Could you check a few things on this model? Use its own coordinates, in mm. Give positions to 0.01 mm unless a question says otherwise; leave off trailing zeros. Write each loop counter-clockwise with the first axis right and the second up, starting at its lowest first coordinate (ties: lowest second). Pieces come first, ordered by that corner, then holes. Notation, with made-up numbers: M 85.25,55 L 110.25,55 A22 ccw 110.25,81 Z; hole C 46.25,64 d2. An arc over 180 degrees is marked long. Write each question's results on one line, items separated by ' | '. Start each with the question number.
from build123d import *

# Parameters (mm, degrees)
F0_R     = 1.7272
F1_DEPTH = 3.175


with BuildPart() as f1:
    # F0 (on Top) → F1 (new body)
    with BuildSketch(Plane.XY):
        with BuildLine():
            Line((0, 0), (0, -9.525))
            Line((0, -9.525), (55.515764, -9.525))
            Line((55.515764, -9.525), (55.515764, 0))
            Line((55.515764, 0), (30.030001, 11.420443))
            ThreePointArc((30.030001, 11.420443), (27.757882, 11.90625), (25.485763, 11.420443))
            Line((25.485763, 11.420443), (0, 0))
        make_face()
        with Locations((14.2875, -4.7625)):
            Circle(F0_R, mode=Mode.SUBTRACT)
        with Locations((41.228264, -4.7625)):
            Circle(F0_R, mode=Mode.SUBTRACT)
        with Locations((27.757882, 6.35)):
            Circle(F0_R, mode=Mode.SUBTRACT)
    extrude(amount=F1_DEPTH)


solid = f1.part
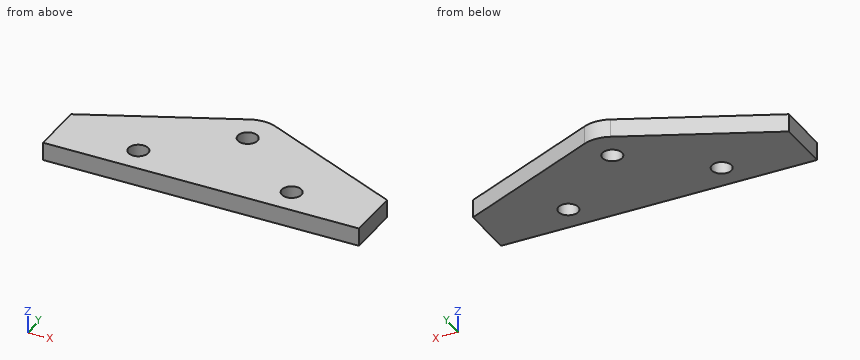
Q1. If we section it at C-C (y = -5.25): Please give me the cut outline in (x, z) (3 decimals).
Q2. I'm going to push a flat-ended pin straight in: P1, Ø1.5, axis at y = 4.5, z = 0.5, coming from the -X side. Where does the tip first touch, or does it pass through?
Q3. If we section it at B-B (z = 0.9): Count the separate pieces of the cut face and the enclosed holes in it, plus the area to 3 significant figures.
Q4. If we section it at D-D (x = 38): Please give me the cut outline in (y, z) (3 decimals).
Q5. If we section it at A-A (y = 7): Please give me the cut outline in (x, z) (3 decimals), plus the area to 3 significant figures.
Q6. Please list where these lines run through material, in increasing order: line 1 (X direction, y = -4.25, z = 2.1); line 2 (X direction, y = 5.25, z = 2.1); line 3 (X direction, y = 6.75, z = 2.8). Write a range as [from, to].
Determined:
1) outline: M 0,0 L 12.631,0 L 12.631,3.175 L 0,3.175 Z; M 15.944,0 L 39.571,0 L 39.571,3.175 L 15.944,3.175 Z; M 42.885,0 L 55.516,0 L 55.516,3.175 L 42.885,3.175 Z
2) P1: stops at x = 8.37
3) separate pieces: 1 | enclosed holes: 3 | area: 845 mm²
4) outline: M -9.525,0 L 7.849,0 L 7.849,3.175 L -9.525,3.175 Z
5) outline: M 15.621,0 L 26.158,0 L 26.158,3.175 L 15.621,3.175 Z; M 29.358,0 L 39.895,0 L 39.895,3.175 L 29.358,3.175 Z | area: 66.9 mm²
6) line 1: x = [0, 12.64], [15.94, 39.58], [42.88, 55.52] | line 2: x = [11.72, 26.43], [29.09, 43.8] | line 3: x = [15.06, 26.08], [29.44, 40.45]
